```python
from build123d import *

# Parameters (mm, degrees)
SKETCH_1_R      = 1.6
SKETCH_1_R_2    = 1.7
SKETCH_1_R_3    = 2.1
SKETCH_1_R_4    = 3.5
EXTRUDE_1_DEPTH = 5


with BuildPart() as part:
    # 草图1 → 凸台-拉伸1 (new body)
    with BuildSketch(Plane(origin=(0, 0, 0), x_dir=(1, 0, 0), z_dir=(0, 1, 0))):
        Polygon((-140, 75), (-140, -75), (140, -75), (140, -5), (120, -5), (120, 75), align=None)
        with Locations(Location((72, -65, 0), (0, 0, 270))):
            Circle(SKETCH_1_R, mode=Mode.SUBTRACT)
        with Locations(Location((135, -65, 0), (0, 0, 270))):
            Circle(SKETCH_1_R, mode=Mode.SUBTRACT)
        with Locations(Location((-110, 24, 0), (0, 0, 270))):
            Circle(SKETCH_1_R_2, mode=Mode.SUBTRACT)
        with Locations(Location((-79, 24, 0), (0, 0, 270))):
            Circle(SKETCH_1_R_2, mode=Mode.SUBTRACT)
        with Locations(Location((-65, 15.5, 0), (0, 0, 270))):
            Circle(SKETCH_1_R_3, mode=Mode.SUBTRACT)
        with Locations(Location((-110, 55, 0), (0, 0, 270))):
            Circle(SKETCH_1_R_2, mode=Mode.SUBTRACT)
        with Locations(Location((-94.5, 39.5, 0), (0, 0, 270))):
            Circle(SKETCH_1_R_4, mode=Mode.SUBTRACT)
        with Locations(Location((-79, 55, 0), (0, 0, 270))):
            Circle(SKETCH_1_R_2, mode=Mode.SUBTRACT)
        with Locations(Location((-65, 40.5, 0), (0, 0, 270))):
            Circle(SKETCH_1_R_3, mode=Mode.SUBTRACT)
        with Locations(Location((45, 15.5, 0), (0, 0, 270))):
            Circle(SKETCH_1_R_3, mode=Mode.SUBTRACT)
        with Locations(Location((59, 24, 0), (0, 0, 270))):
            Circle(SKETCH_1_R_2, mode=Mode.SUBTRACT)
        with Locations(Location((87, 5, 0), (0, 0, 270))):
            Circle(SKETCH_1_R, mode=Mode.SUBTRACT)
        with Locations(Location((90, 24, 0), (0, 0, 270))):
            Circle(SKETCH_1_R_2, mode=Mode.SUBTRACT)
        with Locations(Location((45, 40.5, 0), (0, 0, 270))):
            Circle(SKETCH_1_R_3, mode=Mode.SUBTRACT)
        with Locations(Location((59, 55, 0), (0, 0, 270))):
            Circle(SKETCH_1_R_2, mode=Mode.SUBTRACT)
        with Locations(Location((74.5, 39.5, 0), (0, 0, 270))):
            Circle(SKETCH_1_R_4, mode=Mode.SUBTRACT)
        with Locations(Location((90, 55, 0), (0, 0, 270))):
            Circle(SKETCH_1_R_2, mode=Mode.SUBTRACT)
    extrude(amount=EXTRUDE_1_DEPTH)


solid = part.part
```
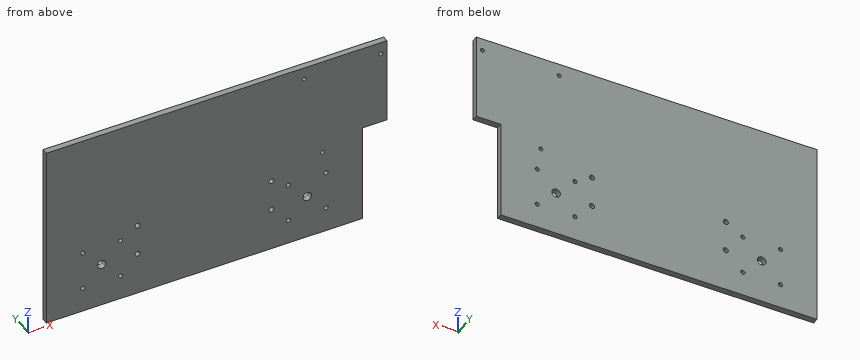
The listing builds one solid part. Answer for the finished solid, in the listing's coordinates (mm). Round coordinates to 2 decimals unless told otherwise and drop trailing zeros. Loops run counter-clockwise (first coordinate to the right, second up) from the corner with the lowest first, then second, coordinate; pieces in that order, holes last.
1) A cutting plane is placed at A-A on y = 2.55. Give the number of separate pieces and of enclosed holes in the cut face, plus the area to 3 significant figures.
Outcome:
separate pieces: 1
enclosed holes: 17
area: 40,200 mm2
2) A cutting plane is placed at B-B on z = -49. Determine the outline of the cut face in (x, y).
Outcome:
outline: (-140, 0) - (120, 0) - (120, 5) - (-140, 5) - close
3) Consider line 1 (X direction, y = 2.65, z = -24); line 2 (X direction, y = 3.1, z = -15.5); line 3 (X direction, y = 3.1, z = 65). Determine where each line is inside the solid, lowest interval first.
Outcome:
line 1: x = -140 to -111.7, -108.3 to -80.7, -77.3 to 57.3, 60.7 to 88.3, 91.7 to 120
line 2: x = -140 to -67.1, -62.9 to 42.9, 47.1 to 120
line 3: x = -140 to 70.4, 73.6 to 133.4, 136.6 to 140
